from build123d import *

# Parameters (mm, degrees)
SKETCH1_W           = 110
SKETCH1_H           = 100
BOSS_EXTRUDE1_DEPTH = 3
SKETCH2_W           = 110
SKETCH2_H           = 100
SKETCH2_W_2         = 104
SKETCH2_H_2         = 94
SKETCH2_R           = 3
BOSS_EXTRUDE2_DEPTH = 7
SKETCH3_R           = 1.5
BOSS_EXTRUDE3_DEPTH = 25
SKETCH5_W           = 20
SKETCH5_H           = 8
BOSS_EXTRUDE4_DEPTH = 10
SKETCH6_W           = 20
SKETCH6_H           = 80
BOSS_EXTRUDE5_DEPTH = 4
FILLET1_R           = 5


with BuildPart() as part:
    # Sketch1 → Boss-Extrude1 (new body)
    with BuildSketch(Plane(origin=(0, 0, 0), x_dir=(1, 0, 0), z_dir=(0, 1, 0))):
        Rectangle(SKETCH1_W, SKETCH1_H)
    extrude(amount=BOSS_EXTRUDE1_DEPTH)

    # Sketch2 → Boss-Extrude2 (add)
    # profile 1 of 5: a face of its own
    with BuildSketch(Plane(origin=(0, 3, 0), x_dir=(1, 0, 0), z_dir=(0, 1, 0))):
        Rectangle(SKETCH2_W, SKETCH2_H)
        Rectangle(SKETCH2_W_2, SKETCH2_H_2, mode=Mode.SUBTRACT)
    # profile 2 of 5: a face of its own
    with BuildSketch(Plane(origin=(0, 3, 0), x_dir=(1, 0, 0), z_dir=(0, 1, 0))):
        with Locations(Location((-41, 35, 0), (0, 0, 270))):
            Circle(SKETCH2_R)
    # profile 3 of 5: a face of its own
    with BuildSketch(Plane(origin=(0, 3, 0), x_dir=(1, 0, 0), z_dir=(0, 1, 0))):
        with Locations(Location((-41, -35, 0), (0, 0, 270))):
            Circle(SKETCH2_R)
    # profile 4 of 5: a face of its own
    with BuildSketch(Plane(origin=(0, 3, 0), x_dir=(1, 0, 0), z_dir=(0, 1, 0))):
        with Locations(Location((41, 35, 0), (0, 0, 270))):
            Circle(SKETCH2_R)
    # profile 5 of 5: a face of its own
    with BuildSketch(Plane(origin=(0, 3, 0), x_dir=(1, 0, 0), z_dir=(0, 1, 0))):
        with Locations(Location((41, -35, 0), (0, 0, 90))):
            Circle(SKETCH2_R)
    extrude(amount=BOSS_EXTRUDE2_DEPTH)

    # Sketch3 → Boss-Extrude3 (add)
    with BuildSketch(Plane(origin=(0, 10, 0), x_dir=(1, 0, 0), z_dir=(0, 1, 0))):
        with Locations(Location((-41, 35, 0), (0, 0, 270))):
            Circle(SKETCH3_R)
        with Locations(Location((41, 35, 0), (0, 0, 270))):
            Circle(SKETCH3_R)
        with Locations(Location((41, -35, 0), (0, 0, 270))):
            Circle(SKETCH3_R)
        with Locations(Location((-41, -35, 0), (0, 0, 270))):
            Circle(SKETCH3_R)
    extrude(amount=BOSS_EXTRUDE3_DEPTH)

    # Sketch5 → Boss-Extrude4 (add)
    with BuildSketch(Plane.XZ):
        with Locations((-30, -36)):
            Rectangle(SKETCH5_W, SKETCH5_H)
        with Locations((-30, 36)):
            Rectangle(SKETCH5_W, SKETCH5_H)
        with Locations((30, 36)):
            Rectangle(SKETCH5_W, SKETCH5_H)
        with Locations((30, -36)):
            Rectangle(SKETCH5_W, SKETCH5_H)
    extrude(amount=BOSS_EXTRUDE4_DEPTH)

    # Sketch6 → Boss-Extrude5 (add)
    with BuildSketch(Plane.XZ.offset(10)):
        with Locations((-30, 0)):
            Rectangle(SKETCH6_W, SKETCH6_H)
        with Locations((30, 0)):
            Rectangle(SKETCH6_W, SKETCH6_H)
    extrude(amount=BOSS_EXTRUDE5_DEPTH)

    # Fillet1
    # the kernel refuses this fillet: 5 mm, written as the material it takes off along each edge
    with BuildSketch(Plane(origin=(-40, -14, -52.5), x_dir=(1, 0, 0), z_dir=(0, 0, 1)), Plane(origin=(-20, -14, 52.5), x_dir=(-1, 0, 0), z_dir=(0, 0, -1)), Plane(origin=(20, -14, -52.5), x_dir=(1, 0, 0), z_dir=(0, 0, 1)), Plane(origin=(40, -14, 52.5), x_dir=(-1, 0, 0), z_dir=(0, 0, -1))) as fillet1_piece_1:
        with BuildLine():
            CenterArc((FILLET1_R, FILLET1_R), FILLET1_R, 180, 90)
            Line((0, FILLET1_R), (0, 0))
            Line((0, 0), (FILLET1_R, 0))
        make_face()
    extrude(amount=105, mode=Mode.SUBTRACT)
    with BuildSketch(Plane(origin=(7.5, -14, 40), x_dir=(0, 0, -1), z_dir=(1, 0, 0)), Plane(origin=(-52.5, -14, 40), x_dir=(0, 0, -1), z_dir=(1, 0, 0))) as fillet1_piece_2:
        with BuildLine():
            CenterArc((FILLET1_R, FILLET1_R), FILLET1_R, 180, 90)
            Line((0, FILLET1_R), (0, 0))
            Line((0, 0), (FILLET1_R, 0))
        make_face()
    extrude(amount=45, mode=Mode.SUBTRACT)
    with BuildSketch(Plane(origin=(52.5, -14, -40), x_dir=(0, 1, 0), z_dir=(-1, 0, 0)), Plane(origin=(-7.5, -14, -40), x_dir=(0, 1, 0), z_dir=(-1, 0, 0))) as fillet1_piece_3:
        with BuildLine():
            CenterArc((FILLET1_R, -FILLET1_R), FILLET1_R, 90, 90)
            Line((0, -FILLET1_R), (0, 0))
            Line((0, 0), (FILLET1_R, 0))
        make_face()
    extrude(amount=45, mode=Mode.SUBTRACT)


solid = part.part
Source: CAD feature listing. Evaluate the final solid. Frame: model axes, mm. A direction names the side the tool comes from. Round coordinates to 2 decimals unless told otherwise and drop trailing zeros. Loops run counter-clockwise (first coordinate to the right, second up) from the corner with the lowest first, then second, coordinate; pieces in that order, holes last. Notation, with made-up numbers: (10.5, 29.5) - (20.5, 29.5) arc R25 cw to (20.5, 66.5) - close; hole circle Ø11 at (26, 82). An arc over 180 degrees is marked (long way). Write item = value, one per line. Start each with the question number.
(1) Set-up query: faces 5 (the face through (40, -4, -36)), 6 (the face through (-30, -4, 40)), 7 (the face through (-30, -4, -40)), 8 (the face through (-52, 6, 1)). Return all of +Z, -Z, +X, -X, +Y, -Y with unobstructed straight access to the full face (end or side cutting, diameter ignored); none if empty.
(2) Pin query (flat end, axial travel): pin 1 (4 mm diameter, centred on y = -3, z = 34, fed in from -X); pin 2 (10 mm diameter, centred on x = -9, z = -13.5, fed in from -Y); pin 3 (4 mm diameter, centred on y = -5, z = -36.5, fed in from +X). Return the tip coordinate at first contact, or that it passes through.
(3) Section query A-A, the plane y = -5. Output: boundary loops of the cut face in (x, z), plus the area to 3 significant figures.
(4) Section query B-B, the plane z = 8. Output: boundary loops of the cut face in (x, y), plus the area to 3 significant figures.
(5) Ray query, line 1 along X through (y, z) = (7.5, -10); line 2 along Y through (x, z) = (-26.5, 11); line 3 along Z through (x, y) = (9, 7). Return the intervals inside material, ascending. Write a range as from..to.
(6) Section query C-C, the plane x = -48. Output: boundary loops of the cut face in (y, z).
(7) Section query D-D, the plane y = 26. Output: boundary loops of the cut face in (x, z), plus the area to 3 significant figures.
(8) Pull-direction query (X, two-part tool) for faces 1 (the face through (-42.3, 10, -33.7)), 2 (the face through (30, -12, 39)), 3 (the face through (40.1, 22.3, 33.8)), 4 (the face through (40, -4, 36)); classes: +X half, -X half, draft (parallel to the pull), parting line (faces both ways), or undercut.
Conclusion:
q1.face_5 = +Z, -Z, +X, -Y
q1.face_6 = +Z, +X, -X, -Y
q1.face_7 = -Z, +X, -X, -Y
q1.face_8 = +Y
q2.pin_1 = -40
q2.pin_2 = 0
q2.pin_3 = 40
q3.outline = (-40, -40) - (-20, -40) - (-20, -32) - (-40, -32) - close; (-40, 32) - (-20, 32) - (-20, 40) - (-40, 40) - close; (20, -40) - (40, -40) - (40, -32) - (20, -32) - close; (20, 32) - (40, 32) - (40, 40) - (20, 40) - close
q3.area = 640 mm2
q4.outline = (-55, 0) - (55, 0) - (55, 10) - (52, 10) - (52, 3) - (-52, 3) - (-52, 10) - (-55, 10) - close; (-39.9, -10) arc R5 ccw to (-35, -14) - (-25, -14) arc R5 ccw to (-20.1, -10) - close; (20.1, -10) arc R5 ccw to (25, -14) - (35, -14) arc R5 ccw to (39.9, -10) - close
q4.area = 511 mm2
q5.line_1 = -55..-52, 52..55
q5.line_2 = -14..-10, 0..3
q5.line_3 = -50..-47, 47..50
q6.outline = (0, -50) - (10, -50) - (10, -47) - (3, -47) - (3, 47) - (10, 47) - (10, 50) - (0, 50) - close
q7.outline = circle Ø3 at (-41, -35); circle Ø3 at (-41, 35); circle Ø3 at (41, -35); circle Ø3 at (41, 35)
q7.area = 28.3 mm2
q8.face_1 = undercut
q8.face_2 = draft
q8.face_3 = undercut
q8.face_4 = +X half
